from build123d import *

# Parameters (mm, degrees)
F2_R      = 25
F1_R      = 60
F5_R      = 42.5
F3_FACE_R = 60
F9_R      = 55
F7_R      = 20
F8_R      = 37.5
F12_R     = 8
F13_R     = 42.5
F14_DEPTH = 5
F15_R     = 10


with BuildPart() as f3:
    # F2 (on offset) → F3 section 0
    with BuildSketch(Plane.XY.offset(50)):
        Circle(F2_R)
    # F1 (on Top) → F3 section 1
    with BuildSketch(Plane.XY):
        Circle(F1_R)
    loft()

    # F5 (on offset) → F6 section 0
    with BuildSketch(Plane.XY.offset(-60)):
        Circle(F5_R)
    # F3_face (on face) → F6 section 1
    with BuildSketch(Plane(origin=(0, 0, 0), x_dir=(1, 0, 0), z_dir=(0, 0, -1))):
        Circle(F3_FACE_R)
    loft()

    # F9 (on Top) → F10 section 0
    with BuildSketch(Plane.XY):
        Circle(F9_R)
    # F7 (on offset) → F10 section 1
    with BuildSketch(Plane.XY.offset(50)):
        Circle(F7_R)
    loft(mode=Mode.SUBTRACT)

    # F8 (on offset) → F11 section 0
    with BuildSketch(Plane.XY.offset(-60)):
        Circle(F8_R)
    # F9 (on Top) → F11 section 1
    with BuildSketch(Plane.XY):
        Circle(F9_R)
    loft(mode=Mode.SUBTRACT)

    # F12
    f12_edges = [f3.edges().sort_by_distance(p)[0] for p in [
        (-60, 0, 0),
    ]]
    fillet(f12_edges, radius=F12_R)

    # F13 (on offset) → F14 (join)
    with BuildSketch(Plane.XY.offset(-60)):
        Circle(F13_R)
    extrude(amount=-F14_DEPTH)

    # F15
    f15_edges = [f3.edges().sort_by_distance(p)[0] for p in [
        (-42.5, 0, -60),
    ]]
    fillet(f15_edges, radius=F15_R)


solid = f3.part
The listing builds one solid part. Answer for the finished solid, in the listing's coordinates (mm). A direction names the side the tool comes from. Round coordinates to 2 decimals unless told otherwise and drop trailing zeros. Order: outer loops, then holes, each group sorted by start corner. A loop starts at its lowest first (then second) coordinate and runs counter-clockwise, first axis right, second up. Notation, with made-up numbers: (88, -8) -> (133, -8) arc R14 ccw to (133, 19) -> close; hole circle Ø7 at (70, 86). An arc over 180 degrees is marked (long way). Write each question's results on one line, items separated by ' | '. Start each with the question number.
Q1. Find section A-A (z = 31.5). Determine the outline of the cut face in (x, y), then the cut area to 3 significant figures.
Q2. Each of these flat-tipped pins is pushed along its axis until it touches: pin 1 (10 mm diameter, centred on y = 20.5, z = -41.5, fed in from -X); pin 2 (2 mm diameter, centred on y = 36.5, z = -2.5, fed in from -X); pin 3 (6 mm diameter, centred on x = 19.5, y = -43.5, fed in from +Z). Where does it stop, or does it pass through?
Q3. Find section B-B (z = -14.5). Determine the outline of the cut face in (x, y).
Q4. Which of the six approach directions +Z, -Z, +X, -X, +Y, -Y give full straight-line access (tool end or side, diameter ignored) to faces 5 (the conical face through (-9.21, -41.473, -42.913)), 6 (the cylindrical face through (-33.727, -25.861, -63.189)), 7 (the flat face through (-11, 17, 50))?
Q5. The mould has two halves that part along Z. Classify faces 1 (the conical face through (-5.5, -25, 42)), 2 (the flat face through (-1, 1, -60)), 3 (the conical face through (25.8, 8.13, 47.07)), 4 (the flat face through (-1, 1, -65)): pulls with the +Z half, pulls with the -Z half, needs draft (parallel to the pull), parting line crosses it, or undercut.
Q6. Straight lines are drawn through the part: probe 1 along Y at (x, z) = (-3, -50); probe 2 along Y at (x, z) = (32.5, -33.5); probe 3 along X at (y, z) = (2, 5). For each, find the intervals that lie inside material, in ascending order. Write a range as from..to.
Worked answers:
1) outline: circle Ø75.9 at (0, 0); hole circle Ø65.9 at (0, 0) | area: 1,110 mm2
2) pin 1: stops at x = -45.9 | pin 2: stops at x = -47.36 | pin 3: stops at z = 21.9
3) outline: circle Ø111.54 at (0, 0); hole circle Ø101.54 at (0, 0)
4) face 5: none | face 6: -Z | face 7: +Z, +X, -X, +Y, -Y
5) face 1: undercut | face 2: undercut | face 3: pulls with the +Z half | face 4: pulls with the -Z half
6) probe 1: y = -45.32..-40.31, 40.31..45.32 | probe 2: y = -38.3..-31.46, 31.46..38.3 | probe 3: x = -56.46..-51.46, 51.46..56.46
